The listing builds one solid part. Answer for the finished solid, in the listing's coordinates (mm). Face numbers are marked on the shaded views. A direction names the side the tool comes from. Round coordinates to 2 decimals unless told otherwise and drop trailing zeros. Write each loop counter-clockwise with the first axis right and the second up, starting at its lowest first coordinate (ties: lowest second). Pieces come first, ordered by that corner, then holes.
(1) A cutting plane is placed at A-A, the plane y = -2. Give the vertices of the cut face in (x, z).
(2) The mould has two halves that part along X. Classify the marked faces 1, 2 and 3: +X half, -X half, draft (parallel to the pull), parting line (faces both ways), or undercut.
(3) For the marked faces 4, 5, 6 and 7, determine the directions among +Z, -Z, +X, -X, +Y, -Y from which every point of the face is accessible in a straight line to the end or side of a thin tool.
(4) Find the intervals of material crossed by probe 1 along Y at (x, z) = (-20, 5); probe 2 along Y at (x, z) = (1, 5.75); probe 3 along X at (y, z) = (2, 5.5), in increasing order.
(5) A cutting plane is placed at B-B, the plane x = -8. Give the vertices of the cut face in (y, z).
(6) A cutting plane is placed at C-C, the plane y = 10. Give the vertices of the cut face in (x, z), and give its area (3 significant figures).
(7) Each of these flat-tipped pins is pushed along its axis until it touches: pin 1 Ø2.5 at (x, z) = (32.5, 6.5) entering from +Y; pin 2 Ø2.5 at (y, z) = (-33, 4) entering from -X; pin 3 Ø2.5 at (y, z) = (-32, 4) entering from +X. Where does it stop, or does it pass through?
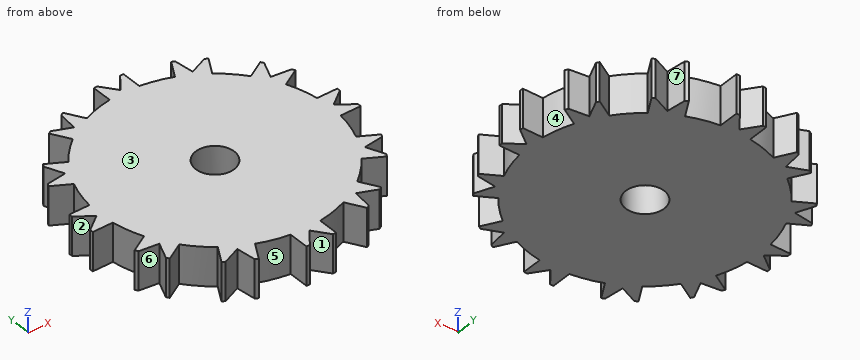
Autodesk Fusion 360 part; units mm, degrees
sketch "turn wheel" plane through (0, 0, 0) normal (0, 0, 1) x (1, 0, 0)
  circle A0 centre (0, 0) radius 30
  line L0 (-3.8635, 29.7502) -> (-3.8635, 35)
  line L1 (-3.8635, 35) -> (-3, 35)
  line L2 (-3, 35) -> (0, 31)
  line L3 (0, 35) -> (0, 30) construction
  line L4 (3.8635, 29.7502) -> (3.8635, 35)
  line L5 (3.8635, 35) -> (3, 35)
  line L6 (3, 35) -> (0, 31)
  line L7 (-18.2209, 23.8327) -> (-20.8458, 28.3792)
  line L8 (-20.0981, 28.8109) -> (-15.5, 26.8468)
  line L9 (-20.8458, 28.3792) -> (-20.0981, 28.8109)
  line L10 (-14.9019, 31.8109) -> (-15.5, 26.8468)
  line L11 (-14.1542, 32.2426) -> (-14.9019, 31.8109)
  line L12 (-11.5292, 27.6961) -> (-14.1542, 32.2426)
  line L13 (-27.6961, 11.5292) -> (-32.2426, 14.1542)
  line L14 (-31.8109, 14.9019) -> (-26.8468, 15.5)
  line L15 (-32.2426, 14.1542) -> (-31.8109, 14.9019)
  line L16 (-28.8109, 20.0981) -> (-26.8468, 15.5)
  line L17 (-28.3792, 20.8458) -> (-28.8109, 20.0981)
  line L18 (-23.8327, 18.2209) -> (-28.3792, 20.8458)
  line L19 (-29.7502, -3.8635) -> (-35, -3.8635)
  line L20 (-35, -3) -> (-31, 0)
  line L21 (-35, -3.8635) -> (-35, -3)
  line L22 (-35, 3) -> (-31, 0)
  line L23 (-35, 3.8635) -> (-35, 3)
  line L24 (-29.7502, 3.8635) -> (-35, 3.8635)
  line L25 (-23.8327, -18.2209) -> (-28.3792, -20.8458)
  line L26 (-28.8109, -20.0981) -> (-26.8468, -15.5)
  line L27 (-28.3792, -20.8458) -> (-28.8109, -20.0981)
  line L28 (-31.8109, -14.9019) -> (-26.8468, -15.5)
  line L29 (-32.2426, -14.1542) -> (-31.8109, -14.9019)
  line L30 (-27.6961, -11.5292) -> (-32.2426, -14.1542)
  line L31 (-11.5292, -27.6961) -> (-14.1542, -32.2426)
  line L32 (-14.9019, -31.8109) -> (-15.5, -26.8468)
  line L33 (-14.1542, -32.2426) -> (-14.9019, -31.8109)
  line L34 (-20.0981, -28.8109) -> (-15.5, -26.8468)
  line L35 (-20.8458, -28.3792) -> (-20.0981, -28.8109)
  line L36 (-18.2209, -23.8327) -> (-20.8458, -28.3792)
  line L37 (3.8635, -29.7502) -> (3.8635, -35)
  line L38 (3, -35) -> (0, -31)
  line L39 (3.8635, -35) -> (3, -35)
  line L40 (-3, -35) -> (0, -31)
  line L41 (-3.8635, -35) -> (-3, -35)
  line L42 (-3.8635, -29.7502) -> (-3.8635, -35)
  line L43 (18.2209, -23.8327) -> (20.8458, -28.3792)
  line L44 (20.0981, -28.8109) -> (15.5, -26.8468)
  line L45 (20.8458, -28.3792) -> (20.0981, -28.8109)
  line L46 (14.9019, -31.8109) -> (15.5, -26.8468)
  line L47 (14.1542, -32.2426) -> (14.9019, -31.8109)
  line L48 (11.5292, -27.6961) -> (14.1542, -32.2426)
  line L49 (27.6961, -11.5292) -> (32.2426, -14.1542)
  line L50 (31.8109, -14.9019) -> (26.8468, -15.5)
  line L51 (32.2426, -14.1542) -> (31.8109, -14.9019)
  line L52 (28.8109, -20.0981) -> (26.8468, -15.5)
  line L53 (28.3792, -20.8458) -> (28.8109, -20.0981)
  line L54 (23.8327, -18.2209) -> (28.3792, -20.8458)
  line L55 (29.7502, 3.8635) -> (35, 3.8635)
  line L56 (35, 3) -> (31, 0)
  line L57 (35, 3.8635) -> (35, 3)
  line L58 (35, -3) -> (31, 0)
  line L59 (35, -3.8635) -> (35, -3)
  line L60 (29.7502, -3.8635) -> (35, -3.8635)
  line L61 (23.8327, 18.2209) -> (28.3792, 20.8458)
  line L62 (28.8109, 20.0981) -> (26.8468, 15.5)
  line L63 (28.3792, 20.8458) -> (28.8109, 20.0981)
  line L64 (31.8109, 14.9019) -> (26.8468, 15.5)
  line L65 (32.2426, 14.1542) -> (31.8109, 14.9019)
  line L66 (27.6961, 11.5292) -> (32.2426, 14.1542)
  line L67 (11.5292, 27.6961) -> (14.1542, 32.2426)
  line L68 (14.9019, 31.8109) -> (15.5, 26.8468)
  line L69 (14.1542, 32.2426) -> (14.9019, 31.8109)
  line L70 (20.0981, 28.8109) -> (15.5, 26.8468)
  line L71 (20.8458, 28.3792) -> (20.0981, 28.8109)
  line L72 (18.2209, 23.8327) -> (20.8458, 28.3792)
  dimension "d1" = 60
  dimension "d2" = 5.2498
  dimension "d3" = 0.8635
  dimension "d4" = 5
  dimension "d6" = 360
extrude "Extrude1" add sketch "turn wheel" along normal blind 10
sketch "hole punch" plane through (0, 0, 10) normal (0, 0, 1) x (-1, 0, 0)
  arc A0 (-23.8327, -18.2209) -> (-18.2209, -23.8327) centre (0, 0) ccw
  line L0 (-18.2209, -23.8327) -> (-20.8458, -28.3792)
  line L1 (-20.8458, -28.3792) -> (-20.0981, -28.8109)
  line L2 (-20.0981, -28.8109) -> (-15.5, -26.8468)
  line L3 (-15.5, -26.8468) -> (-14.9019, -31.8109)
  line L4 (-14.9019, -31.8109) -> (-14.1542, -32.2426)
  line L5 (-14.1542, -32.2426) -> (-11.5292, -27.6961)
  arc A1 (-11.5292, -27.6961) -> (-3.8635, -29.7502) centre (0, 0) ccw
  line L6 (-3.8635, -29.7502) -> (-3.8635, -35)
  line L7 (-3.8635, -35) -> (-3, -35)
  line L8 (-3, -35) -> (0, -31)
  line L9 (0, -31) -> (3, -35)
  line L10 (3, -35) -> (3.8635, -35)
  line L11 (3.8635, -35) -> (3.8635, -29.7502)
  arc A2 (3.8635, -29.7502) -> (11.5292, -27.6961) centre (0, 0) ccw
  line L12 (11.5292, -27.6961) -> (14.1542, -32.2426)
  line L13 (14.1542, -32.2426) -> (14.9019, -31.8109)
  line L14 (14.9019, -31.8109) -> (15.5, -26.8468)
  line L15 (15.5, -26.8468) -> (20.0981, -28.8109)
  line L16 (20.0981, -28.8109) -> (20.8458, -28.3792)
  line L17 (20.8458, -28.3792) -> (18.2209, -23.8327)
  arc A3 (18.2209, -23.8327) -> (23.8327, -18.2209) centre (0, 0) ccw
  line L18 (23.8327, -18.2209) -> (28.3792, -20.8458)
  line L19 (28.3792, -20.8458) -> (28.8109, -20.0981)
  line L20 (28.8109, -20.0981) -> (26.8468, -15.5)
  line L21 (26.8468, -15.5) -> (31.8109, -14.9019)
  line L22 (31.8109, -14.9019) -> (32.2426, -14.1542)
  line L23 (32.2426, -14.1542) -> (27.6961, -11.5292)
  arc A4 (27.6961, -11.5292) -> (29.7502, -3.8635) centre (0, 0) ccw
  line L24 (29.7502, -3.8635) -> (35, -3.8635)
  line L25 (35, -3.8635) -> (35, -3)
  line L26 (35, -3) -> (31, 0)
  line L27 (31, 0) -> (35, 3)
  line L28 (35, 3) -> (35, 3.8635)
  line L29 (35, 3.8635) -> (29.7502, 3.8635)
  arc A5 (29.7502, 3.8635) -> (27.6961, 11.5292) centre (0, 0) ccw
  line L30 (27.6961, 11.5292) -> (32.2426, 14.1542)
  line L31 (32.2426, 14.1542) -> (31.8109, 14.9019)
  line L32 (31.8109, 14.9019) -> (26.8468, 15.5)
  line L33 (26.8468, 15.5) -> (28.8109, 20.0981)
  line L34 (28.8109, 20.0981) -> (28.3792, 20.8458)
  line L35 (28.3792, 20.8458) -> (23.8327, 18.2209)
  arc A6 (23.8327, 18.2209) -> (18.2209, 23.8327) centre (0, 0) ccw
  line L36 (18.2209, 23.8327) -> (20.8458, 28.3792)
  line L37 (20.8458, 28.3792) -> (20.0981, 28.8109)
  line L38 (20.0981, 28.8109) -> (15.5, 26.8468)
  line L39 (15.5, 26.8468) -> (14.9019, 31.8109)
  line L40 (14.9019, 31.8109) -> (14.1542, 32.2426)
  line L41 (14.1542, 32.2426) -> (11.5292, 27.6961)
  arc A7 (11.5292, 27.6961) -> (3.8635, 29.7502) centre (0, 0) ccw
  line L42 (3.8635, 29.7502) -> (3.8635, 35)
  line L43 (3.8635, 35) -> (3, 35)
  line L44 (3, 35) -> (0, 31)
  line L45 (0, 31) -> (-3, 35)
  line L46 (-3, 35) -> (-3.8635, 35)
  line L47 (-3.8635, 35) -> (-3.8635, 29.7502)
  arc A8 (-3.8635, 29.7502) -> (-11.5292, 27.6961) centre (0, 0) ccw
  line L48 (-11.5292, 27.6961) -> (-14.1542, 32.2426)
  line L49 (-14.1542, 32.2426) -> (-14.9019, 31.8109)
  line L50 (-14.9019, 31.8109) -> (-15.5, 26.8468)
  line L51 (-15.5, 26.8468) -> (-20.0981, 28.8109)
  line L52 (-20.0981, 28.8109) -> (-20.8458, 28.3792)
  line L53 (-20.8458, 28.3792) -> (-18.2209, 23.8327)
  arc A9 (-18.2209, 23.8327) -> (-23.8327, 18.2209) centre (0, 0) ccw
  line L54 (-23.8327, 18.2209) -> (-28.3792, 20.8458)
  line L55 (-28.3792, 20.8458) -> (-28.8109, 20.0981)
  line L56 (-28.8109, 20.0981) -> (-26.8468, 15.5)
  line L57 (-26.8468, 15.5) -> (-31.8109, 14.9019)
  line L58 (-31.8109, 14.9019) -> (-32.2426, 14.1542)
  line L59 (-32.2426, 14.1542) -> (-27.6961, 11.5292)
  arc A10 (-27.6961, 11.5292) -> (-29.7502, 3.8635) centre (0, 0) ccw
  line L60 (-29.7502, 3.8635) -> (-35, 3.8635)
  line L61 (-35, 3.8635) -> (-35, 3)
  line L62 (-35, 3) -> (-31, 0)
  line L63 (-31, 0) -> (-35, -3)
  line L64 (-35, -3) -> (-35, -3.8635)
  line L65 (-35, -3.8635) -> (-29.7502, -3.8635)
  arc A11 (-29.7502, -3.8635) -> (-27.6961, -11.5292) centre (0, 0) ccw
  line L66 (-27.6961, -11.5292) -> (-32.2426, -14.1542)
  line L67 (-32.2426, -14.1542) -> (-31.8109, -14.9019)
  line L68 (-31.8109, -14.9019) -> (-26.8468, -15.5)
  line L69 (-26.8468, -15.5) -> (-28.8109, -20.0981)
  line L70 (-28.8109, -20.0981) -> (-28.3792, -20.8458)
  line L71 (-28.3792, -20.8458) -> (-23.8327, -18.2209)
  line L72 (31, 0) -> (-31, 0) construction
  line L73 (0, -31) -> (0, 31) construction
  circle A12 centre (0, 0) radius 5
extrude "Extrude2" cut sketch "hole punch" against normal blind 10 contours A12
Solutions:
1. outline: (-33.67, 0) - (-4.58, 0) - (-4.58, 10) - (-33.67, 10) - close; (4.58, 0) - (33.67, 0) - (33.67, 10) - (4.58, 10) - close
2. face 1: undercut
2. face 2: -X half
2. face 3: draft
3. face 4: +Z, -Z, +X
3. face 5: +Z, -Z, -Y
3. face 6: +Z, -Z, -X
3. face 7: +Z, -Z, +Y
4. probe 1: y = -28.77 to -26.91, -22.36 to 22.36, 26.91 to 28.77
4. probe 2: y = -32.33 to -4.9, 4.9 to 32.33
4. probe 3: x = -33.67 to -4.58, 4.58 to 33.67
5. outline: (-28.91, 0) - (28.91, 0) - (28.91, 10) - (-28.91, 10) - close
6. outline: (-28.28, 0) - (28.28, 0) - (28.28, 10) - (-28.28, 10) - close
6. area: 566 mm2
7. pin 1: stops at y = 14.97
7. pin 2: stops at x = -14.91
7. pin 3: stops at x = 15.03
